from build123d import *

# Parameters (mm, degrees)
SKETCH1_W           = 321
SKETCH1_H           = 220
BOSS_EXTRUDE1_DEPTH = 1
SKETCH2_R           = 8.25
CUT_EXTRUDE1_DEPTH  = 195.579675198
SKETCH3_R           = 3
CUT_EXTRUDE2_DEPTH  = 195.579675198


with BuildPart() as part:
    # Sketch1 → Boss-Extrude1 (new body)
    with BuildSketch(Plane.YZ):
        Rectangle(SKETCH1_W, SKETCH1_H)
    extrude(amount=BOSS_EXTRUDE1_DEPTH)

    # Sketch2 → Cut-Extrude1 (cut, through all)
    with BuildSketch(Plane.YZ.offset(1)):
        with Locations(Location((-75, 50, 0), (0, 0, 270))):
            Circle(SKETCH2_R)
        with Locations(Location((-25, 50, 0), (0, 0, 270))):
            Circle(SKETCH2_R)
        with Locations(Location((25, 50, 0), (0, 0, 270))):
            Circle(SKETCH2_R)
        with Locations(Location((75, 50, 0), (0, 0, 270))):
            Circle(SKETCH2_R)
        with Locations(Location((-25, 0, 0), (0, 0, 270))):
            Circle(SKETCH2_R)
        with Locations(Location((25, 0, 0), (0, 0, 270))):
            Circle(SKETCH2_R)
        with Locations(Location((75, 0, 0), (0, 0, 270))):
            Circle(SKETCH2_R)
        with Locations(Location((-25, -50, 0), (0, 0, 270))):
            Circle(SKETCH2_R)
        with Locations(Location((25, -50, 0), (0, 0, 270))):
            Circle(SKETCH2_R)
        with Locations(Location((75, -50, 0), (0, 0, 270))):
            Circle(SKETCH2_R)
        with Locations(Location((-75, 0, 0), (0, 0, 270))):
            Circle(SKETCH2_R)
        with Locations(Location((-75, -50, 0), (0, 0, 270))):
            Circle(SKETCH2_R)
    extrude(amount=-CUT_EXTRUDE1_DEPTH, mode=Mode.SUBTRACT)

    # Sketch3 → Cut-Extrude2 (cut, through all)
    with BuildSketch(Plane.YZ.offset(1)):
        with Locations(Location((-150.5, 100, 0), (0, 0, 270))):
            Circle(SKETCH3_R)
        with Locations(Location((150.5, 100, 0), (0, 0, 90))):
            Circle(SKETCH3_R)
        with Locations(Location((-150.5, -100, 0), (0, 0, 90))):
            Circle(SKETCH3_R)
        with Locations(Location((150.5, -100, 0), (0, 0, 270))):
            Circle(SKETCH3_R)
    extrude(amount=-CUT_EXTRUDE2_DEPTH, mode=Mode.SUBTRACT)


solid = part.part
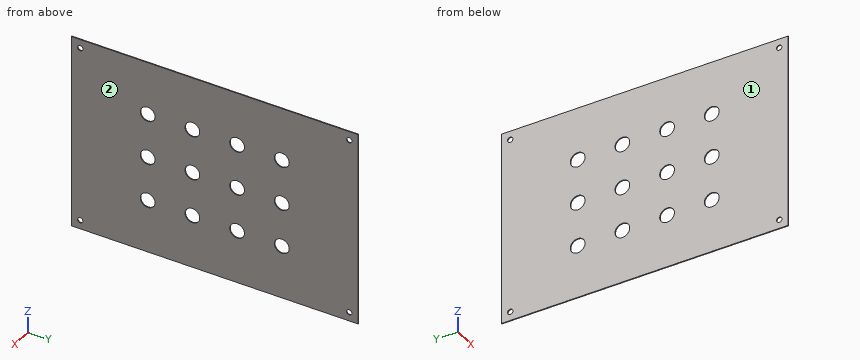
Build history of the part. All positions in model axes, mm. Face numbers are marked on the shaded views. Round coordinates to 2 decimals unless told otherwise and drop trailing zeros. Write each loop counter-clockwise with the first axis right and the second up, starting at its lowest first coordinate (ties: lowest second). Pieces come first, ordered by that corner, then holes. Notation, with made-up numbers: (54, 15) -> (66, 15) arc R11 ccw to (66, 28) -> close; hole circle Ø6 at (65.5, 22). An arc over 180 degrees is marked (long way). Write item = value, one per line.
(1) Band-saw the part on D-D (z = -45.5). Give the cut face in (x, y), then the cut area to 3 significant figures.
Answer:
outline = (0, -160.5) -> (1, -160.5) -> (1, -81.91) -> (0, -81.91) -> close; (0, -68.09) -> (1, -68.09) -> (1, -31.91) -> (0, -31.91) -> close; (0, -18.09) -> (1, -18.09) -> (1, 18.09) -> (0, 18.09) -> close; (0, 31.91) -> (1, 31.91) -> (1, 68.09) -> (0, 68.09) -> close; (0, 81.91) -> (1, 81.91) -> (1, 160.5) -> (0, 160.5) -> close
area = 266 mm2
(2) Two-plate mould, pull along X, no slides. Class the marked faces 1 and 2: pulls with the +X half, pulls with the -X half, needs draft (parallel to the pull), parting line crosses it, or undercut.
Answer:
face_1 = pulls with the -X half
face_2 = pulls with the +X half
(3) Band-saw the part on A-A (y = -75). Give the cut face in (x, z), then the cut area to 4 significant figures.
Answer:
outline = (0, -110) -> (1, -110) -> (1, -58.25) -> (0, -58.25) -> close; (0, -41.75) -> (1, -41.75) -> (1, -8.25) -> (0, -8.25) -> close; (0, 8.25) -> (1, 8.25) -> (1, 41.75) -> (0, 41.75) -> close; (0, 58.25) -> (1, 58.25) -> (1, 110) -> (0, 110) -> close
area = 170.5 mm2
(4) Band-saw the part on C-C (z = 0). Give the cut face in (x, y), then the cut area to 3 significant figures.
Answer:
outline = (0, -160.5) -> (1, -160.5) -> (1, -83.25) -> (0, -83.25) -> close; (0, -66.75) -> (1, -66.75) -> (1, -33.25) -> (0, -33.25) -> close; (0, -16.75) -> (1, -16.75) -> (1, 16.75) -> (0, 16.75) -> close; (0, 33.25) -> (1, 33.25) -> (1, 66.75) -> (0, 66.75) -> close; (0, 83.25) -> (1, 83.25) -> (1, 160.5) -> (0, 160.5) -> close
area = 255 mm2
(5) Band-saw the part on B-B (x = 0.6). State how many separate pieces and enclosed holes the cut face has, then the cut area to 3 significant figures.
Answer:
separate_pieces = 1
enclosed_holes = 16
area = 67,900 mm2
(6) Probe L1, parallel to Y at x = 0.65, z = 49.5; L2, parallel to Z at x = 0.75, y = 81. List the from-to ranges inside material, lowest first.
Answer:
L1 = -160.5 to -83.23, -66.77 to -33.23, -16.77 to 16.77, 33.23 to 66.77, 83.23 to 160.5
L2 = -110 to -55.66, -44.34 to -5.66, 5.66 to 44.34, 55.66 to 110
